from build123d import *

# Parameters (mm, degrees)
F1_R     = 1.5
F1_W     = 3.125
F1_H     = 20
F2_DEPTH = 3.125


with BuildPart() as f2:
    # F1 (on Front) → F2 (new body)
    with BuildSketch(Plane.XZ):
        Polygon((-35, -25), (0, -25), (35, -25), (35, -10), (31.875, -10), (31.875, 5), (35, 5), (35, 20), (31.875, 20), (31.875, 35), (35, 35), (35, 50), (31.875, 50), (31.875, 65), (35, 65), (35, 80), (35, 95), (31.875, 95), (31.875, 110), (35, 110), (35, 125), (31.875, 125), (31.875, 140), (35, 140), (35, 155), (31.875, 155), (31.875, 170), (35, 170), (35, 185), (0, 185), (-35, 185), (-35, 170), (-31.875, 170), (-31.875, 155), (-35, 155), (-35, 140), (-31.875, 140), (-31.875, 125), (-35, 125), (-35, 110), (-31.875, 110), (-31.875, 95), (-35, 95), (-35, 80), (-35, 65), (-31.875, 65), (-31.875, 50), (-35, 50), (-35, 35), (-31.875, 35), (-31.875, 20), (-35, 20), (-35, 5), (-31.875, 5), (-31.875, -10), (-35, -10), align=None)
        with Locations((-25, 0)):
            Circle(F1_R, mode=Mode.SUBTRACT)
        with Locations((25, 0)):
            Circle(F1_R, mode=Mode.SUBTRACT)
        with Locations((-30, 80)):
            Rectangle(F1_W, F1_H, mode=Mode.SUBTRACT)
        with Locations((-25, 160)):
            Circle(F1_R, mode=Mode.SUBTRACT)
        with Locations((30, 80)):
            Rectangle(F1_W, F1_H, mode=Mode.SUBTRACT)
        with Locations((25, 160)):
            Circle(F1_R, mode=Mode.SUBTRACT)
    extrude(amount=F2_DEPTH)


solid = f2.part
Work out the finished part from the listing and answer in its coordinate system (mm). Round coordinates to 2 decimals unless told otherwise and drop trailing zeros. Loops run counter-clockwise (first coordinate to the right, second up) from the corner with the lowest first, then second, coordinate; pieces in that order, holes last. Notation, with made-up numbers: (67, 61.5) - (95, 61.5) arc R26 cw to (95, 76.5) - close; hole circle Ø6 at (16.5, 27). An arc over 180 degrees is marked (long way). Use one line per item in the form item = value. Start each with the question number.
(1) Find section B-B on y = -1.7. Give the number of separate pieces and of enclosed holes in the cut face, and give its area (3 significant figures).
(2) Flat-ended cylindrical pins translate along their axes: P1, Ø0.9, axis at y = -1.5, z = 54, coming from the +X side (3 decimals); P2, Ø1.6, axis at y = -1.5, z = -5.5, coming from the -X side (3 decimals). Find the tip coordinate at first contact, or state that the pin passes through.
(3) Find section A-A on z = 101. Determine the outline of the cut face in (x, y) (3 decimals), and give its area (3 significant figures).
(4) Consider line 1 (X direction, y = -1.4, z = 160) (3 decimals); line 2 (Z direction, x = -25, y = -1.2); line 3 (Z direction, x = 31, y = -0.5). Determine where each line is inside the solid, lowest interval first.
Answer list:
q1.separate_pieces = 1
q1.enclosed_holes = 6
q1.area = 14,000 mm^2
q2.P1 = 31.875
q2.P2 = -31.875
q3.outline = (-31.875, -3.125) - (31.875, -3.125) - (31.875, 0) - (-31.875, 0) - close
q3.area = 199 mm^2
q4.line_1 = -31.875 to -26.5, -23.5 to 23.5, 26.5 to 31.875
q4.line_2 = -25 to -1.5, 1.5 to 158.5, 161.5 to 185
q4.line_3 = -25 to 70, 90 to 185
